Solid Edge part; units mm, degrees
sketch "Sketch1" plane through (0, 0, 0) normal (0, 0, 1) x (1, 0, 0)
  arc A0 (5.888, 58.8462) -> (5.888, 1.1538) centre (153.0882, 30) ccw
  arc A1 (-5.888, 58.8462) -> (-5.888, 1.1538) centre (-153.0882, 30) cw
  arc A2 (5.888, 1.1538) -> (-5.888, 1.1538) centre (0, 0) cw
  arc A3 (-5.888, 58.8462) -> (5.888, 58.8462) centre (0, 60) cw
extrude "Protrusion1" add sketch "Sketch1" along normal blind 6
sketch "Sketch2" plane through (0, 30, 6) normal (0, 0, 1) x (1, 0, 0)
  circle A0 centre (0, -30) radius 4
  circle A1 centre (0, 30) radius 4
extrude "VaciadoExtruido_1" cut sketch "Sketch2" against normal blind 5
hole "Agujero_1" at (0, 60, 1) direction (0, 0, -1) diameter 3.5 end up to next
hole "Hole1" at (0, 0, 1) direction (0, 0, -1) diameter 3.5 end up to next
chamfer "Chaflán_1" distance 0.5 angle 45 10 edges at (3.0882, 30, 6) (0, -6, 6) (-3.0882, 30, 6) (0, 66, 6) (3.0882, 30, 0) (0, -6, 0) (-3.0882, 30, 0) (0, 66, 0) (-4, 0, 6) (-4, 60, 6)
For this review, take the finished solid that the model builds, in its own axes (mm). A direction names the side the tool comes from. Round coordinates to 2 decimals unless told otherwise and drop trailing zeros. Loops run counter-clockwise (first coordinate to the right, second up) from the corner with the lowest first, then second, coordinate; pieces in that order, holes last.
(1) We need section B-B (z = 3.6). Give the boundary of the cut face in (x, y), plus the area to 3 significant figures.
Returned:
outline: (-5.89, 1.15) arc R6 ccw (long way) to (5.89, 1.15) arc R150 cw to (5.89, 58.85) arc R6 ccw (long way) to (-5.89, 58.85) arc R150 cw to start; hole circle Ø8 at (0, 0); hole circle Ø8 at (0, 60)
area: 504 mm2
(2) Mouldability with a two-part tool opening along X and no side actions: class faces 3 (the cylindrical face through (0, -6, 3)), 4 (the flat face through (0, 30, 0)), 5 (the cylindrical face through (-0.67, -1.617, 0.507)), 6 (the cylindrical face through (-3.09, 30.41, 2.96)) as released by +X, released by -X, zero draft, split by the parting line, or undercut.
Returned:
face 3: split by the parting line
face 4: zero draft
face 5: undercut
face 6: released by -X
(3) Tool access review of faces 1 (the cylindrical face through (-0.867, 56.095, 3.282)), 2 (the cylindrical face through (3.09, 29.59, 2.96)): name each direction out of +Z, -Z, +X, -X, +Y, -Y from which nothing blocks a thin tool from reaching the whole face with its end or side.
Returned:
face 1: +Z
face 2: +Z, -Z, +X
(4) Wall thickness on line 1 along Y through (x, z) = (0, 2.7); line 2 along X through (y, z) = (60, 0.8); line 3 along Y through (x, z) = (-1.75, 1.2): over which ranges is each line inside the solid? List them lowest first.
Returned:
line 1: y = -6 to -4, 4 to 56, 64 to 66
line 2: x = -6 to -1.75, 1.75 to 6
line 3: y = -5.74 to -3.6, 3.6 to 56.4, 63.6 to 65.74
(5) We need section C-C (x = 0). Give the boundary of the cut face in (y, z).
Returned:
outline: (-6, 0.5) - (-5.5, 0) - (-1.75, 0) - (-1.75, 1) - (-4, 1) - (-4, 5.5) - (-4.5, 6) - (-5.5, 6) - (-6, 5.5) - close; (1.75, 0) - (58.25, 0) - (58.25, 1) - (56, 1) - (56, 5.5) - (55.5, 6) - (4.5, 6) - (4, 5.5) - (4, 1) - (1.75, 1) - close; (61.75, 0) - (65.5, 0) - (66, 0.5) - (66, 5.5) - (65.5, 6) - (64.5, 6) - (64, 5.5) - (64, 1) - (61.75, 1) - close
(6) Clearance check with flat-ended pins moving along their axes: P1, Ø4, axis at x = -1, y = 62, coming from the +Z side; P2, Ø4, axis at x = 0, y = 60, coming from the +Z side; P3, Ø2, axis at x = 0, y = 0, coming from the -Z side; P4, Ø2, axis at x = 4, y = 39, coming from the +Z side. State where each tip first meets the part, or that it passes through.
Returned:
P1: stops at z = 5.74
P2: stops at z = 1
P3: passes through
P4: stops at z = 5.86
(7) We need section A-A (y = 60). Give the boundary of the cut face in (x, z), plus the area to 4 significant figures.
Returned:
outline: (-6, 0.5) - (-5.5, 0) - (-1.75, 0) - (-1.75, 1) - (-4, 1) - (-4, 5.5) - (-4.5, 6) - (-5.5, 6) - (-6, 5.5) - close; (1.75, 0) - (5.5, 0) - (6, 0.5) - (6, 5.5) - (5.5, 6) - (4.5, 6) - (4, 5.5) - (4, 1) - (1.75, 1) - close
area: 27.75 mm2
